CAD build for the part. Positions are in the model's coordinates, mm. A direction names the side the tool comes from. Give positions to 0.01 mm unless a question says otherwise; leave off trailing zeros. Write each loop counter-clockwise with the first axis right and the second up, starting at its lowest first coordinate (ties: lowest second). Pieces come first, ordered by that corner, then holes. Notation, with made-up numbers: (71, 10.5) - (129, 10.5) arc R24 ccw to (129, 34.5) - close; hole circle Ø6 at (48, 66). An arc over 180 degrees is marked (long way). Put each result on its own line as item: value. Start each with the question number.
1. Wall check: line 1 (Z direction, x = 26, y = 3.3); line 2 (X direction, y = -10, z = -6.5); line 3 (X direction, y = 4, z = 9). Give the ranges that are in metal, low to high.
2. Tool access for faces 3 (the flat face through (26, 2, 16)), 4 (the conical face through (17.19, 40.15, -5.41)), 5 (the cylindrical face through (-27.15, 2.96, 11.77)), 6 (the cylindrical face through (12.5, 15.1, -0.3)), 7 (the flat face through (-26, 2, 16)): list every direction of +Z, -Z, +X, -X, +Y, -Y with a clear straight run to the whole face (end or side of a thin tool).
3. Cut at B-B on x = 0. Give the number of separate pieces and of enclosed holes in the cut face, and give its area (3 significant figures).
4. Cut at A-A on y = 2.5. List the corners of the cut face in (x, z).
5. Mould opens along Y. For faces 1 (the flat face through (8.4, 51.25, 8.9)), 2 (the flat face through (-26, 2, -16)) say: +Y half, -Y half, draft (parallel to the pull), parting line (faces both ways), or undercut.
6. Cut at C-C on y = -15. List the corners of the cut face in (x, z), and give its area (3 significant figures).
7. Drop flat-ended pins along their axis: pin 1 (8 mm diameter, centred on x = -15, y = 15, fed in from -Z); pin 2 (2 mm diameter, centred on x = 26, y = 3, fed in from +Z); pin 3 (1 mm diameter, centred on y = -3.5, z = 16.5, fed in from -X). Give the stop position or say it passes through.
from build123d import *

# Parameters (mm, degrees)
SKETCH1_W               = 40
SKETCH1_H               = 40
SKETCH1_R               = 2.5
SKETCH1_R_2             = 16
BOSS_EXTRUDE2_DEPTH     = 20
FILLET2_R               = 3
SKETCH3_W               = 18
SKETCH3_H               = 3
LPATTERN1_COUNT         = 5
LPATTERN1_PITCH         = 5.25
CUT_EXTRUDE2_REACH      = 97.226
CUT_EXTRUDE2_END_RADIUS = 16
SKETCH6_R               = 10
SKETCH7_W               = 12
SKETCH7_H               = 32
SKETCH7_R               = 3
BOSS_EXTRUDE4_DEPTH     = 6
FILLET3_R               = 1.5


with BuildPart() as part:
    # Sketch1 → Boss-Extrude2 (new, symmetric)
    with BuildSketch(Plane.XY):
        Rectangle(SKETCH1_W, SKETCH1_H)
        with Locations((-15, 15)):
            Circle(SKETCH1_R, mode=Mode.SUBTRACT)
        with Locations((15, 15)):
            Circle(SKETCH1_R, mode=Mode.SUBTRACT)
        with Locations((15, -15)):
            Circle(SKETCH1_R, mode=Mode.SUBTRACT)
        with Locations((-15, -15)):
            Circle(SKETCH1_R, mode=Mode.SUBTRACT)
        Circle(SKETCH1_R_2, mode=Mode.SUBTRACT)
    extrude(amount=BOSS_EXTRUDE2_DEPTH, both=True)

    # Fillet2
    fillet2_edges = [part.edges().sort_by_distance(p)[0] for p in [
        (20, -20, 0),
        (-20, -20, 0),
        (-20, 20, 0),
        (20, 20, 0),
    ]]
    fillet(fillet2_edges, radius=FILLET2_R)

    # Sketch2 → Revolve1 (revolve)
    with BuildSketch(Plane.XY, mode=Mode.PRIVATE) as revolve1_sk:
        Polygon((0, 20), (0, 70), (-22, 70), (-18, 40), (-15, 40), (-15, 20), align=None)
    revolve(revolve1_sk.sketch.rotate(Axis((0, 20, 0), (0, 1, 0)), 180), axis=Axis((0, 20, 0), (0, 1, 0)))

    # Sketch3 → Cut-Revolve1 (revolve, cut)
    with BuildSketch(Plane.XY, mode=Mode.PRIVATE) as cut_revolve1_sk:
        with Locations((-21, 44.5)):
            Rectangle(SKETCH3_W, SKETCH3_H)
    cut_revolve1 = revolve(cut_revolve1_sk.sketch.rotate(Axis((0, 34.204860636, 0), (0, 1, 0)), 270), axis=Axis((0, 34.204860636, 0), (0, 1, 0)), mode=Mode.SUBTRACT)

    # LPattern1: Cut-Revolve1 ×5
    with Locations(*[(0, i * LPATTERN1_PITCH, 0) for i in range(1, LPATTERN1_COUNT)]):
        add(cut_revolve1, mode=Mode.SUBTRACT)

    # Cut-Extrude2: up to this cylinder (the profile starts outside it)
    cut_extrude2_end = Plane(origin=(0, 0, 0), z_dir=(0, 0, -1)) * Cylinder(CUT_EXTRUDE2_END_RADIUS, 227.452, mode=Mode.PRIVATE)
    # Sketch6 → Cut-Extrude2 (cut, up to the surface)
    with BuildSketch(Plane(origin=(0, 70, 0), x_dir=(1, 0, 0), z_dir=(0, 1, 0)), mode=Mode.PRIVATE) as cut_extrude2_sk1:
        with Locations(Location((0, 0, 0), (0, 0, 180))):
            Circle(SKETCH6_R)
    cut_extrude2_tool1 = extrude(cut_extrude2_sk1.sketch, amount=-CUT_EXTRUDE2_REACH, mode=Mode.PRIVATE) - cut_extrude2_end
    add(cut_extrude2_tool1.solids().sort_by_distance((0, 70, 0))[0], mode=Mode.SUBTRACT)

    # Sketch7 → Boss-Extrude4 (add)
    with BuildSketch(Plane(origin=(0, 0, 0), x_dir=(1, 0, 0), z_dir=(0, 1, 0))):
        with Locations((-26, 0)):
            Rectangle(SKETCH7_W, SKETCH7_H)
        with Locations(Location((-26, 9, 0), (0, 0, 270))):
            Circle(SKETCH7_R, mode=Mode.SUBTRACT)
        with Locations(Location((-26, -9, 0), (0, 0, 270))):
            Circle(SKETCH7_R, mode=Mode.SUBTRACT)
    boss_extrude4 = extrude(amount=BOSS_EXTRUDE4_DEPTH)

    # Mirror1: Boss-Extrude4 across plane
    add(boss_extrude4.mirror(Plane(origin=(0, 0, 0), x_dir=(0, 0, 1), z_dir=(1, 0, 0))))

    # Fillet3
    fillet3_edges = [part.edges().sort_by_distance(p)[0] for p in [
        (-20, 6, 0),
        (-26, 6, -16),
        (-32, 6, 0),
        (-26, 6, 16),
        (-20, 3, 16),
        (-20, 3, -16),
        (-32, 3, -16),
        (-32, 3, 16),
        (20, 6, 0),
        (20, 3, -16),
        (26, 6, 16),
        (20, 3, 16),
        (32, 6, 0),
        (32, 3, 16),
        (26, 6, -16),
        (32, 3, -16),
        (-15, 20, 0),
    ]]
    fillet(fillet3_edges, radius=FILLET3_R)


solid = part.part
Report:
1. line 1: z = -16 to -12, -6 to 6, 12 to 16
1. line 2: x = -20 to -12.49, 12.49 to 20
1. line 3: x = -32 to -29, -23 to -15.49, 15.49 to 23, 29 to 32
2. face 3: +Z, +X, +Y, -Y
2. face 4: none
2. face 5: +Y, -Y
2. face 6: +Z, -Z
2. face 7: +Z, -X, +Y, -Y
3. separate pieces: 3
3. enclosed holes: 0
3. area: 801 mm²
4. outline: (-32, -14.5) arc R1.5 ccw to (-30.5, -16) - (-21.5, -16) arc R1.5 cw to (-20, -17.5) - (-20, -20) - (-15.8, -20) - (-15.8, 20) - (-20, 20) - (-20, 17.5) arc R1.5 cw to (-21.5, 16) - (-30.5, 16) arc R1.5 ccw to (-32, 14.5) - close; (15.8, -20) - (20, -20) - (20, -17.5) arc R1.5 cw to (21.5, -16) - (30.5, -16) arc R1.5 ccw to (32, -14.5) - (32, 14.5) arc R1.5 ccw to (30.5, 16) - (21.5, 16) arc R1.5 cw to (20, 17.5) - (20, 20) - (15.8, 20) - close; hole circle Ø6 at (-26, -9); hole circle Ø6 at (-26, 9); hole circle Ø6 at (26, -9); hole circle Ø6 at (26, 9)
5. face 1: undercut
5. face 2: draft
6. outline: (-20, -20) - (-17.5, -20) - (-17.5, 20) - (-20, 20) - close; (-12.5, -20) - (-5.57, -20) - (-5.57, 20) - (-12.5, 20) - close; (5.57, -20) - (12.5, -20) - (12.5, 20) - (5.57, 20) - close; (17.5, -20) - (20, -20) - (20, 20) - (17.5, 20) - close
6. area: 755 mm²
7. pin 1: stops at z = -20
7. pin 2: stops at z = 16
7. pin 3: stops at x = -20
